Read the model definition and answer for the solid it produces. Units are mm, in the model's axes. A direction names the side the tool comes from. Give positions to 0.01 mm unless a question says otherwise; leave off trailing zeros. Order: outer loops, then holes, each group sorted by start corner. A loop starts at its lowest first (then second) coordinate and runs counter-clockwise, first axis right, second up. Notation, with made-up numbers: (7, 44.25) - (23, 44.25) arc R18 cw to (23, 70.25) - close; hole circle Ø4 at (43, 75). An arc over 180 degrees is marked (long way). Write each question's results on one line, items separated by ' | '.
Autodesk Inventor part; units mm, degrees
ref_plane "YZ Plane" through (0, 0, 0) normal (1, 0, 0) x (0, 1, 0)
ref_plane "XZ Plane" through (0, 0, 0) normal (0, 1, 0) x (-1, 0, 0)
ref_plane "XY Plane" through (0, 0, 0) normal (0, 0, 1) x (1, 0, 0)
sketch "Sketch1" plane through (0, 0, 0) normal (0, 1, 0) x (-1, 0, 0)
  line L0 (-152.4, 152.4) -> (152.4, 152.4)
  line L1 (152.4, 152.4) -> (152.4, -152.4)
  line L2 (152.4, -152.4) -> (-152.4, -152.4)
  line L3 (-152.4, -152.4) -> (-152.4, 152.4)
  line L4 (-152.4, 152.4) -> (152.4, -152.4) construction
  line L5 (152.4, 152.4) -> (-152.4, -152.4) construction
  line L6 (0, -35) -> (-30.3109, -17.5)
  line L7 (-30.3109, -17.5) -> (-30.3109, 17.5)
  line L8 (-30.3109, 17.5) -> (0, 35)
  line L9 (0, 35) -> (30.3109, 17.5)
  line L10 (30.3109, 17.5) -> (30.3109, -17.5)
  line L11 (30.3109, -17.5) -> (0, -35)
  arc A0 (54.3646, 35.4255) -> (35.7748, 54.1354) centre (0, 0) ccw construction
  arc A1 (61.905, 40.339) -> (40.7367, 61.6439) centre (0, 0) ccw
  arc A2 (46.8242, 30.5119) -> (30.8128, 46.6268) centre (0, 0) ccw
  arc A3 (46.8242, 30.5119) -> (61.905, 40.339) centre (54.3646, 35.4255) ccw
  arc A4 (40.7367, 61.6439) -> (30.8128, 46.6268) centre (35.7748, 54.1354) ccw
  arc A5 (-61.6439, 40.7367) -> (-46.6268, 30.8128) centre (-54.1354, 35.7748) ccw
  arc A6 (-30.5119, 46.8242) -> (-46.6268, 30.8128) centre (0, 0) ccw
  arc A7 (-40.339, 61.905) -> (-61.6439, 40.7367) centre (0, 0) ccw
  arc A8 (-30.5119, 46.8242) -> (-40.339, 61.905) centre (-35.4255, 54.3646) ccw
  arc A9 (-40.7367, -61.6439) -> (-30.8128, -46.6268) centre (-35.7748, -54.1354) ccw
  arc A10 (-46.8242, -30.5119) -> (-30.8128, -46.6268) centre (0, 0) ccw
  arc A11 (-61.905, -40.339) -> (-40.7367, -61.6439) centre (0, 0) ccw
  arc A12 (-46.8242, -30.5119) -> (-61.905, -40.339) centre (-54.3646, -35.4255) ccw
  arc A13 (61.6439, -40.7367) -> (46.6268, -30.8128) centre (54.1354, -35.7748) ccw
  arc A14 (30.5119, -46.8242) -> (46.6268, -30.8128) centre (0, 0) ccw
  arc A15 (40.339, -61.905) -> (61.6439, -40.7367) centre (0, 0) ccw
  arc A16 (30.5119, -46.8242) -> (40.339, -61.905) centre (35.4255, -54.3646) ccw
  circle A17 centre (0, 0) radius 7.5
  dimension "d1" = 304.8
  dimension "d2" = 304.8
  dimension "d5" = 35
  dimension "d11" = 360
  dimension "d13" = 18
  dimension "d14" = 15
extrude "Extrusion1" add sketch "Sketch1" along normal blind 5 contours L0 L1 L2 L3 | L6 L7 L8 L9 L10 L11
chamfer "Chamfer1" distance 38.1 angle 45 4 edges at (152.4, 2.5, -152.4) (-152.4, 2.5, -152.4) (-152.4, 2.5, 152.4) (152.4, 2.5, 152.4)
ref_plane "Work Plane1" through (0, 0, -17.5) normal (1, 0, 0) x (0, 0, -1)
properties part number "bottom plate"
(1) Section B-B (x = 0) is taken. Give the vertices of the cut face in (y, z).
Conclusion:
outline: (0, -152.4) - (5, -152.4) - (5, -7.5) - (0, -7.5) - close; (0, 7.5) - (5, 7.5) - (5, 152.4) - (0, 152.4) - close
(2) Section D-D (z = 131) is taken. Give the vertices of the cut face in (x, y).
Conclusion:
outline: (-135.7, 0) - (135.7, 0) - (135.7, 5) - (-135.7, 5) - close
(3) Section A-A (y = 2.35) is taken. Give the vertices of the cut face in (x, z) (3 decimals), plus the area to 3 significant figures.
Conclusion:
outline: (-152.4, -114.3) - (-114.3, -152.4) - (114.3, -152.4) - (152.4, -114.3) - (152.4, 114.3) - (114.3, 152.4) - (-114.3, 152.4) - (-152.4, 114.3) - close; hole (-61.905, 40.339) arc R9 ccw to (-46.824, 30.512) arc R55.889 cw to (-30.813, 46.627) arc R9 ccw to (-40.737, 61.644) arc R73.886 ccw to start; hole (-61.644, -40.737) arc R73.886 ccw to (-40.339, -61.905) arc R9 ccw to (-30.512, -46.824) arc R55.889 cw to (-46.627, -30.813) arc R9 ccw to start; hole circle Ø15 at (0, 0); hole (30.512, 46.824) arc R55.889 cw to (46.627, 30.813) arc R9 ccw to (61.644, 40.737) arc R73.886 ccw to (40.339, 61.905) arc R9 ccw to start; hole (30.813, -46.627) arc R9 ccw to (40.737, -61.644) arc R73.886 ccw to (61.905, -40.339) arc R9 ccw to (46.824, -30.512) arc R55.889 cw to start | area: 86,900 mm^2
(4) For faces 4 (the face through (-39.505, 2.465, -39.533)), 5 (the face through (133.1, 2.5, -133.6)), determine the directions among +Z, -Z, +X, -X, +Y, -Y from which every point of the face is accessible in a straight line to the end or side of a thin tool.
Conclusion:
face 4: +Y, -Y | face 5: -Z, +X, +Y, -Y
(5) Consider probe 1 along Z at (x, y) = (-61.5, 4); probe 2 along Z at (x, y) = (0, 2.3); probe 3 along X at (y, z) = (1.6, -39). Determine where each line is inside the solid, lowest interval first. Write a range as [from, to].
Conclusion:
probe 1: [-152.4, -40.95], [-30.6, 29.94], [40.95, 152.4] | probe 2: [-152.4, -7.5], [7.5, 152.4] | probe 3: [-152.4, -62.54], [-40.03, 40.03], [62.62, 152.4]
(6) Section C-C (z = 0) is taken. Give the vertices of the cut face in (x, y), plus the area to 3 significant figures.
Conclusion:
outline: (-152.4, 0) - (-7.5, 0) - (-7.5, 5) - (-152.4, 5) - close; (7.5, 0) - (152.4, 0) - (152.4, 5) - (7.5, 5) - close | area: 1,450 mm^2
(7) The mould has two halves that part along X. Classify faces 1 (the face through (-32, 5, 2)), 2 (the face through (-52.228, 2.465, -52.265)), 3 (the face through (-133.1, 2.5, -133.6)): pulls with the +X half, pulls with the -X half, needs draft (parallel to the pull), parting line crosses it, or undercut.
Conclusion:
face 1: needs draft | face 2: undercut | face 3: pulls with the -X half
